from build123d import *

# Parameters (mm, degrees)
BOSS_EXTRUDE1_DEPTH     = 230
CUT_EXTRUDE2_DEPTH      = 93
SKETCH4_W               = 125
SKETCH4_H               = 36.3
CUT_EXTRUDE3_DEPTH      = 18.9
FILLET3_R               = 10
FILLET4_R               = 6
SKETCH5_W               = 22
SKETCH5_H               = 10.18
CUT_EXTRUDE4_DEPTH      = 18.9
CUT_EXTRUDE5_REACH      = 14.9
CUT_EXTRUDE6_REACH      = 232
SKETCH7_R               = 1.65
CUT_EXTRUDE7_DEPTH      = 49
SKETCH9_W               = 3
SKETCH9_H               = 129.384798753
CUT_EXTRUDE8_DEPTH      = 1
CUT_EXTRUDE8_DEPTH_BACK = 5
SKETCH10_W              = 7
SKETCH10_H              = 13.446036232
CUT_EXTRUDE9_DEPTH      = 8
FILLET5_R               = 3


with BuildPart() as part:
    # Sketch1 → Boss-Extrude1 (new body)
    with BuildSketch(Plane.XY):
        Polygon((0, 0), (-8.900488428, -19.193232029), (-8.900488428, -58.18), (8.999511572, -58.18), (8.999511572, -19.193232029), align=None)
    extrude(amount=BOSS_EXTRUDE1_DEPTH)

    # Sketch3 → Cut-Extrude2 (cut)
    with BuildSketch(Plane(origin=(0, 0, 0), x_dir=(-1, 0, 0), z_dir=(0, 0, -1))):
        Polygon((-6, -58.18), (-6, -55.18), (-4, -55.18), (-4, -21.88), (-8.999511572, -21.88), (-8.999511572, -58.18), align=None)
        Polygon((6, -55.18), (4, -55.18), (4, -21.88), (8.999511572, -21.88), (8.999511572, -58.18), (6, -58.18), align=None)
    extrude(amount=-CUT_EXTRUDE2_DEPTH, mode=Mode.SUBTRACT)

    # Sketch4 → Cut-Extrude3 (cut, through all)
    with BuildSketch(Plane.ZY.offset(8.900488428)):
        with Locations((145.5, -40.03)):
            Rectangle(SKETCH4_W, SKETCH4_H)
    extrude(amount=-CUT_EXTRUDE3_DEPTH, mode=Mode.SUBTRACT)

    # Fillet3
    fillet3_edges = [part.edges().sort_by_distance(p)[0] for p in [
        (0, -21.88, 83),
    ]]
    fillet(fillet3_edges, radius=FILLET3_R)

    # Fillet4
    fillet4_edges = [part.edges().sort_by_distance(p)[0] for p in [
        (0.049511572, -21.88, 208),
    ]]
    fillet(fillet4_edges, radius=FILLET4_R)

    # Sketch5 → Cut-Extrude4 (cut, through all)
    with BuildSketch(Plane(origin=(8.999511572, 0, 0), x_dir=(0, 0, -1), z_dir=(1, 0, 0))):
        with Locations((-219, -53.09)):
            Rectangle(SKETCH5_W, SKETCH5_H)
    extrude(amount=-CUT_EXTRUDE4_DEPTH, mode=Mode.SUBTRACT)

    # Sketch6 → Cut-Extrude5 (cut, up to next)
    with BuildSketch(Plane(origin=(4, 0, 0), x_dir=(0, 0, -1), z_dir=(1, 0, 0)), mode=Mode.PRIVATE) as cut_extrude5_sk1:
        with BuildLine():
            Line((-66.4, -35.43), (-16.4, -35.43))
            ThreePointArc((-16.4, -35.43), (-13.3, -38.53), (-16.4, -41.63))
            Line((-16.4, -41.63), (-66.4, -41.63))
            ThreePointArc((-66.4, -41.63), (-69.5, -38.53), (-66.4, -35.43))
        make_face()
    cut_extrude5_tool1 = extrude(cut_extrude5_sk1.sketch, amount=-CUT_EXTRUDE5_REACH, mode=Mode.PRIVATE) & part.part
    add(cut_extrude5_tool1.solids().sort_by_distance((4, -38.53, 41.4))[0], mode=Mode.SUBTRACT)

    # Sketch7 → Cut-Extrude6 (cut, up to next)
    with BuildSketch(Plane.XY.offset(230), mode=Mode.PRIVATE) as cut_extrude6_sk1:
        with Locations((0, -38)):
            Circle(SKETCH7_R)
    cut_extrude6_tool1 = extrude(cut_extrude6_sk1.sketch, amount=-CUT_EXTRUDE6_REACH, mode=Mode.PRIVATE) & part.part
    add(cut_extrude6_tool1.solids().sort_by_distance((0, -38, 230))[0], mode=Mode.SUBTRACT)

    # Sketch8 → Cut-Extrude7 (cut, through all)
    with BuildSketch(Plane.XZ.offset(48)):
        Polygon((0, 228), (-6.5, 223.5), (-6.5, 213.5), (6.5, 213.5), (6.5, 223.5), align=None)
    extrude(amount=-CUT_EXTRUDE7_DEPTH, mode=Mode.SUBTRACT)

    # Sketch9 → Cut-Extrude8 (cut, two sides)
    with BuildSketch(Plane.XZ.offset(58.18)) as cut_extrude8_sk:
        with Locations((0, 45.686714954)):
            Rectangle(SKETCH9_W, SKETCH9_H)
    extrude(amount=CUT_EXTRUDE8_DEPTH, mode=Mode.SUBTRACT)
    extrude(cut_extrude8_sk.sketch, amount=-CUT_EXTRUDE8_DEPTH_BACK, mode=Mode.SUBTRACT)

    # Sketch10 → Cut-Extrude9 (cut)
    with BuildSketch(Plane.XZ.offset(58.18)):
        with Locations((0, 83)):
            Rectangle(SKETCH10_W, SKETCH10_H)
    extrude(amount=-CUT_EXTRUDE9_DEPTH, mode=Mode.SUBTRACT)

    # Fillet5
    fillet5_edges = [part.edges().sort_by_distance(p)[0] for p in [
        (3.5, -54.18, 76.276981884),
        (-3.5, -54.18, 76.276981884),
    ]]
    fillet(fillet5_edges, radius=FILLET5_R)


solid = part.part
CAD build for the part. Positions are in the model's coordinates, mm. A direction names the side the tool comes from. Give positions to 0.01 mm unless a question says otherwise; leave off trailing zeros. Write each loop counter-clockwise with the first axis right and the second up, starting at its lowest first coordinate (ties: lowest second). Pieces come first, ordered by that corner, then holes. Notation, with made-up numbers: (10, 15.5) - (32, 15.5) arc R24 ccw to (32, 46.5) - close; hole circle Ø2 at (-14.5, 26). An arc over 180 degrees is marked (long way). Answer as CSV lines item,"result".
Q1. Pull direction Z, two halves, no side cores. Call faces 5 (the face through (1.5, -56, 38)), 6 (the face through (0, -29, 0)), 7 (the face through (0.175, -23.591, 206.196)): released by +Z, released by -Z, zero draft, split by the parting line, or undercut.
Result set:
face 5,"zero draft"
face 6,"released by -Z"
face 7,"undercut"
Q2. 3-axis set-ups, long thin cutter, end or side, ignore diameter. For faces 1 (the face through (-2, -38, 208)), 2 (the face through (0, -30, 213.5)), 3 (the face through (0.1, -38.6, 69.5)), 4 (the face through (0, -48, 212)): which of +Z, -Z, +X, -X, +Y, -Y reach the whole face in a straight line?
Result set:
face 1,"+X, -X, -Y"
face 2,"+Y, -Y"
face 3,"+X, -X"
face 4,"+Z, +X, -X, -Y"
Q3. Flat gauge pins, fed straight in: pin 1 Ø8 at (x, y) = (-0.5, -6) entering from -Z; pin 2 Ø2 at (y, z) = (-25.5, 54.5) entering from -X; pin 3 Ø2.5 at (x, y) = (0, -38) entering from +Z; pin 4 Ø4 at (y, z) = (-56.5, 44) entering from -X. Where does each tip first touch, or does it go through?
Result set:
pin 1,"z = 0"
pin 2,"x = -4"
pin 3,"z = 83"
pin 4,"x = -6"
Q4. Band-saw the part on C-C (z = 188). Give the cut face in (x, y).
Result set:
outline,"(-8.9, -21.88) - (9, -21.88) - (9, -19.19) - (0, 0) - (-8.9, -19.19) - close"
Q5. Band-saw the part on A-A (z = 21). Give the cut face in (x, y), and give its area (3 significant figures).
Result set:
outline,"(-8.9, -21.88) - (-4, -21.88) - (-4, -35.43) - (4, -35.43) - (4, -21.88) - (9, -21.88) - (9, -19.19) - (0, 0) - (-8.9, -19.19) - close; (-6, -58.18) - (-1.5, -58.18) - (-1.5, -53.18) - (1.5, -53.18) - (1.5, -58.18) - (6, -58.18) - (6, -55.18) - (4, -55.18) - (4, -41.63) - (-4, -41.63) - (-4, -55.18) - (-6, -55.18) - close"
area,"458 mm²"
Q6. Band-saw the part on B-B (y = -25). Give the cut face in (x, z), and give its area (3 significant figures).
Result set:
outline,"(-8.9, 207.26) - (9, 207.26) - (9, 230) - (-8.9, 230) - close; (-4, 0) - (4, 0) - (4, 85.74) - (-4, 85.74) - close; hole (-6.5, 213.5) - (6.5, 213.5) - (6.5, 223.5) - (0, 228) - (-6.5, 223.5) - close"
area,"934 mm²"
Q7. Drill centre lines: line 1 (Z direction, x = -0.25, y = -30); line 2 (Z direction, x = 3.75, y = -37); line 3 (Y direction, x = 0, z = 228.35). Where is each one in solid material? Low to high. Write a range as from..to.
Result set:
line 1,"0..83.18, 208..213.5, 227.83..230"
line 2,"0..13.7, 69.1..83, 208..213.5, 225.4..230"
line 3,"-48..-39.65, -36.35..0"
